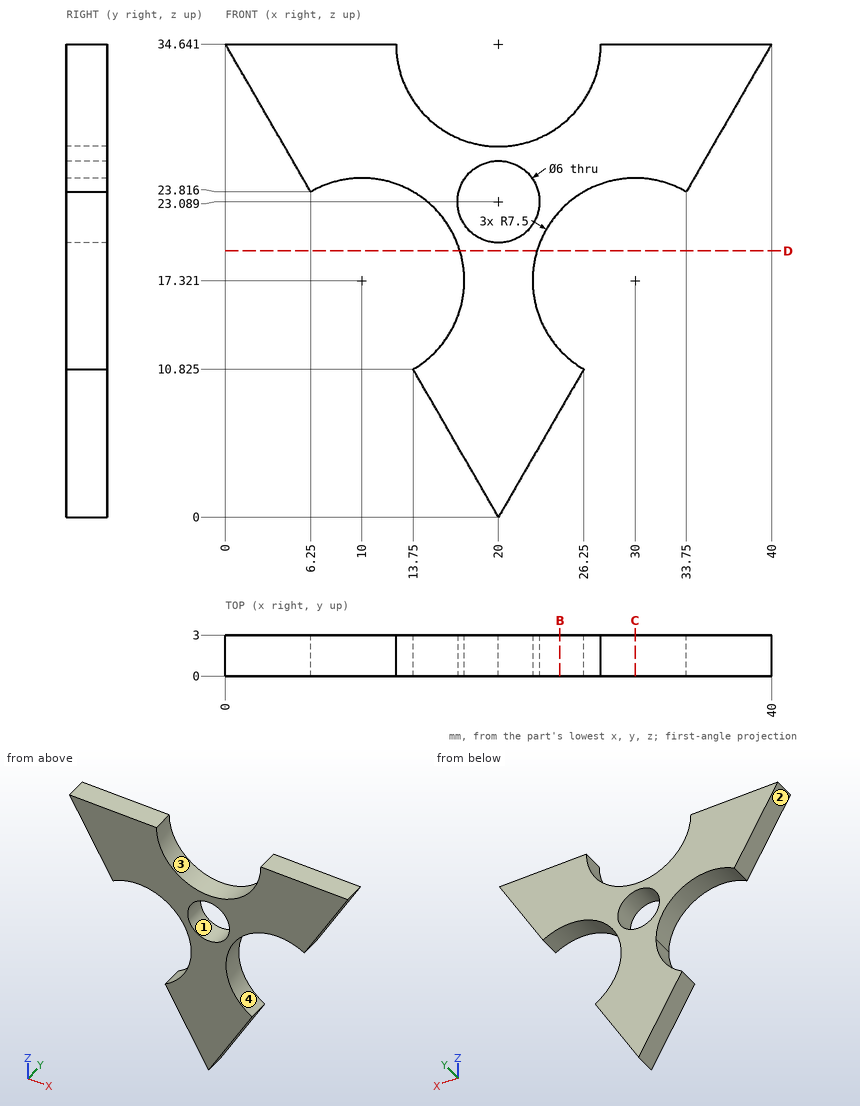
Geometry: see drawing. Coordinates: mm, zero at the bounding-box minimum. Round coordinates to 2 decimals unless told otherwise and drop trailing zeros. Write each loop counter-clockwise with the first axis right and the second up, starting at its lowest first coordinate (ties: lowest second). Pieces come first, ordered by that corner, then holes. Notation, with made-up numbers: M -27.75,58 L 5.25,58 A17 cw 5.25,65 Z; hole C 42.25,69.5 d8. An arc over 180 degrees is marked long. Answer in a Markdown table with one row per item. Add a question column.
(1) Cut plane B-B, the plane x = 24.5. Return the cut outline in (y, z) (1 decimal).
(2) Contact query for a flat-ended pin moving along its axis: pin 1 (3.5 mm diameter, centred on x = 20, z = 23.09, fed in from +Y). Output: stop coordinate, or through.
(3) Cut plane C-C, the plane x = 30. Return the cut outline in (y, z).
(4) Cut plane D-D, the plane z = 19.5. Return the cut outline in (x, y).
(5) Draft query along Z for the marked faces 1, 2, 3 and 4. Return one class per face: pulls with the +Z half, pulls with the -Z half, needs draft (parallel to the pull), parting line crosses it, or undercut.
(6) Ray query, L1, parallel to Z at x = 25.5, y = 1.3 (1 decimal); L2, parallel to X at y = 0.65, z = 31 (1 decimal); L3, parallel to Z at x = 23.5, y = 1.9 (1 decimal). Return the intervals inside material, ascending.
Established:
| question | item | result |
|---|---|---|
| 1 | outline | M 0,7.8 L 3,7.8 L 3,12.2 L 0,12.2 Z; M 0,22.4 L 3,22.4 L 3,28.6 L 0,28.6 Z |
| 2 | pin 1 | through |
| 3 | outline | M 0,24.82 L 3,24.82 L 3,34.64 L 0,34.64 Z |
| 4 | outline | M 17.18,0 L 22.82,0 L 22.82,3 L 17.18,3 Z |
| 5 | face 1 | undercut |
| 5 | face 2 | pulls with the -Z half |
| 5 | face 3 | pulls with the +Z half |
| 5 | face 4 | undercut |
| 6 | L1 | 9.5 to 11.3, 23.3 to 29.5 |
| 6 | L2 | 2.1 to 13.4, 26.6 to 37.9 |
| 6 | L3 | 6.1 to 13.6, 21.1 to 28 |
